Check sheet for the modelled part. Datum: model origin and axes. Units: mm. Round coordinates to 2 decimals unless told otherwise and drop trailing zeros. Order: outer loops, then holes, each group sorted by start corner. A loop starts at its lowest first (then second) coordinate and runs counter-clockwise, first axis right, second up.
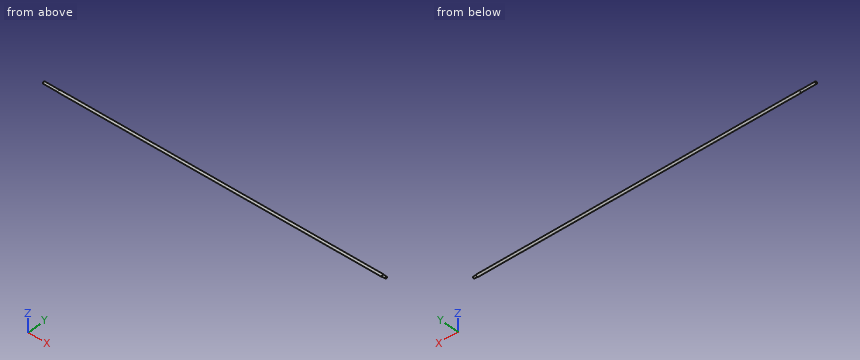
from build123d import *

# Parameters (mm, degrees)
F0_R     = 4
F1_DEPTH = 1097
F2_R     = 3.5
F3_DEPTH = 52
F4_R     = 3
F5_DEPTH = 12
F6_SIZE  = 0.75
F7_SIZE  = 0.75


with BuildPart() as f1:
    # F0 (on Right) → F1 (new body)
    with BuildSketch(Plane.YZ):
        Circle(F0_R)
    extrude(amount=F1_DEPTH)

    # F2 (on Right) → F3 (join)
    with BuildSketch(Plane.YZ):
        Circle(F2_R)
    extrude(amount=-F3_DEPTH)

    # F4 (on face) → F5 (join)
    with BuildSketch(Plane.YZ.offset(1097)):
        Circle(F4_R)
    extrude(amount=F5_DEPTH)

    # F6
    f6_edges = [f1.edges().sort_by_distance(p)[0] for p in [
        (1109, -3, 0),
    ]]
    chamfer(f6_edges, length=F6_SIZE)

    # F7
    f7_edges = [f1.edges().sort_by_distance(p)[0] for p in [
        (-52, -3.5, 0),
    ]]
    chamfer(f7_edges, length=F7_SIZE)


solid = f1.part
1) Sectioned sample at A-A on x = 612. Record the cut outline in (y, z).
2) Scan lines: line 1 (Y direction, x = 642.5, z = 2.25); line 2 (Y direction, x = 675, z = 2.5); line 3 (X direction, y = -3, z = -2). Record each from-to range of solid material in increasing order.
3) Gauge pin test, flat ends, axial feed: pin 1 (3 mm diameter, centred on x = 216, z = -3, fed in from +Y); pin 2 (3 mm diameter, centred on x = 134, z = 2.5, fed in from +Y); pin 3 (1.5 mm diameter, centred on x = 193.5, z = -1, fed in from -Y). Record the tip position at first contact, or that the pin passes through.
Values found:
1. outline: circle Ø8 at (0, 0)
2. line 1: y = -3.31 to 3.31
2. line 2: y = -3.12 to 3.12
2. line 3: x = 0 to 1097
3. pin 1: stops at y = 3.71
3. pin 2: stops at y = 3.87
3. pin 3: stops at y = -3.99
